from build123d import *

# Parameters (mm, degrees)
F2_R     = 13.7
F2_R_2   = 3
F3_DEPTH = 12.45
F1_R     = 13.8
F1_R_2   = 10.8
F4_DEPTH = 45
F6_D     = 4
F6_DEPTH = 13.8010001


with BuildPart() as f3:
    # F2 (on Right) → F3 (new body, symmetric)
    with BuildSketch(Plane.YZ):
        Circle(F2_R)
        Circle(F2_R_2, mode=Mode.SUBTRACT)
    extrude(amount=F3_DEPTH, both=True)

    # F1 (on offset) → F4 (join)
    with BuildSketch(Plane.XZ.offset(50)):
        Circle(F1_R)
        Circle(F1_R_2, mode=Mode.SUBTRACT)
    extrude(amount=-F4_DEPTH)

    # F6 (through all, one way)
    with BuildSketch(Plane.XY):
        with Locations((0, -36)):
            Circle(F6_D / 2)
    extrude(amount=-F6_DEPTH, mode=Mode.SUBTRACT)


solid = f3.part
Can you work these out from the model? Positions are in its coordinate system, mm. A direction names the side the tool comes from. Give positions to 0.01 mm unless a question says otherwise; leave off trailing zeros. Loops run counter-clockwise (first coordinate to the right, second up) from the corner with the lowest first, then second, coordinate; pieces in that order, holes last. Notation, with made-up numbers: M 40.25,51.5 L 57.25,51.5 A24 cw 57.25,78.5 Z; hole C -17.5,56 d9. An arc over 180 degrees is marked long. One line per item, written item: value. Start each with the question number.
1) I'm going to push flat-ended pins straight in: pin 1 (4 mm diameter, centred on x = -5.5, y = -2.5, fed in from -Z); pin 2 (5 mm diameter, centred on y = 6, z = 2.5, fed in from +X); pin 3 (5 mm diameter, centred on x = -1.5, y = 3.5, fed in from +Z). Where does each tip first touch, or does it pass through?
2) Thinking about a two-plate mould opening in Y: for faces 4 (the face through (-12.45, 3.4, 0.2)), 5 (the face through (0, -3, 0)), 6 (the face through (13, -5, 0)), 7 (the face through (1.847, -36.766, -12.184)), which applies, +Y half, -Y half, draft (parallel to the pull), parting line (faces both ways), or undercut?
3) If I drill on line 1 (Z direction, x = -4, y = 0); line 2 (Y direction, x = 0, z = -12.65); line 3 (X direction, y = -28.5, z = 8.25), over which ranges is the centre line in solid material (lowest first)? Write a range as [from, to].
4) If we section it at D-D, the plane y = -10: Write out the boundary of the cut face in (x, z), and give its area (3 significant figures).
5) If we section it at B-B, the plane y = 0: Write out the boundary of the cut face in (x, z).
6) If we section it at A-A, the plane x = 0: Write out the boundary of the cut face in (y, z) (3 decimals).
7) On a 3-axis mill with a long thin cutter (end or side, diameter ignored), from which of +Z, -Z, +X, -X, +Y, -Y can I reach the whole of each face in a straight line? I mean faces 1 (the face through (-13, -5, 0)), 2 (the face through (6.1, -50, -9.1)), 3 (the face through (10.301, -29.505, 3.244)). Say none if no direction works.
8) If we section it at C-C, the plane z = 0: Write out the boundary of the cut face in (x, y), and give its area (3 significant figures).
Completed:
1. pin 1: stops at z = -13.69
1. pin 2: stops at x = 12.45
1. pin 3: stops at z = 13.66
2. face 4: draft
2. face 5: undercut
2. face 6: +Y half
2. face 7: undercut
3. line 1: z = [-13.7, -3], [3, 13.7]
3. line 2: y = [-50, -38], [-34, 5.26]
3. line 3: x = [-11.06, -6.97], [6.97, 11.06]
4. outline: M -12.45,-9.36 L -10.14,-9.36 A13.8 ccw 10.14,-9.36 L 12.45,-9.36 L 12.45,-5.95 A13.8 ccw 12.45,5.95 L 12.45,9.36 L 10.14,9.36 A13.8 ccw -10.14,9.36 L -12.45,9.36 L -12.45,5.95 A13.8 ccw -12.45,-5.95 Z; hole M -5.38,-9.36 A10.8 ccw 5.38,-9.36 Z; hole M -5.38,9.36 L 5.38,9.36 A10.8 ccw Z
4. area: 591 mm^2
5. outline: M -12.45,-13.7 L 12.45,-13.7 L 12.45,-3 L -12.45,-3 Z; M -12.45,3 L 12.45,3 L 12.45,13.7 L -12.45,13.7 Z
6. outline: M -50,-13.8 L -38,-13.8 L -38,-10.8 L -50,-10.8 Z; M -50,10.8 L -8.429,10.8 A13.7 ccw -8.429,-10.8 L -34,-10.8 L -34,-13.8 L -5,-13.8 L -5,-12.755 A13.7 ccw long -5,12.755 L -5,13.8 L -50,13.8 Z; hole C 0,0 d6
7. face 1: +Z, -Z, -X, +Y
7. face 2: +Z, -Z, +X, -X, -Y
7. face 3: -Y
8. outline: M -13.8,-50 L -10.8,-50 L -10.8,-13.7 L 10.8,-13.7 L 10.8,-50 L 13.8,-50 L 13.8,-5 L 12.45,-5 L 12.45,-3 L -12.45,-3 L -12.45,-5 L -13.8,-5 Z; M -12.45,3 L 12.45,3 L 12.45,13.7 L -12.45,13.7 Z
8. area: 774 mm^2
